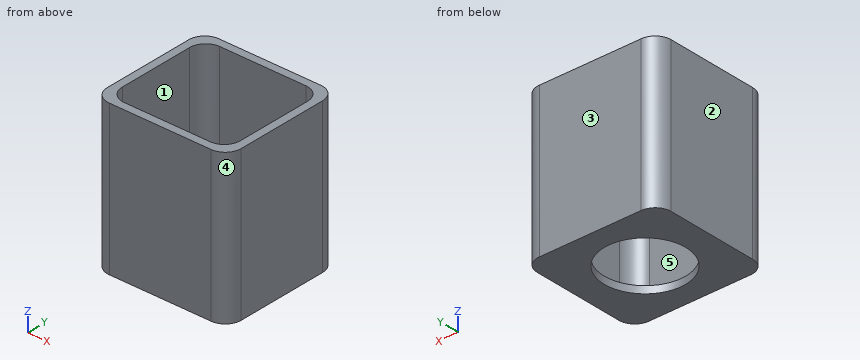
```python
from build123d import *

# Parameters (mm, degrees)
F0_W     = 42
F0_H     = 39
F0_R     = 12.75
F1_DEPTH = 47.25
F2_W     = 37
F2_H     = 34
F2_R     = 12.75
F3_DEPTH = 45
F4_R     = 5


with BuildPart() as f1:
    # F0 (on Top) → F1 (new body)
    with BuildSketch(Plane.XY):
        Rectangle(F0_W, F0_H)
        Circle(F0_R, mode=Mode.SUBTRACT)
    extrude(amount=F1_DEPTH)

    # F2 (on face) → F3 (cut)
    with BuildSketch(Plane.XY.offset(47.25)):
        Rectangle(F2_W, F2_H)
        Circle(F2_R, mode=Mode.SUBTRACT)
    extrude(amount=-F3_DEPTH, mode=Mode.SUBTRACT)

    # F4
    f4_edges = [f1.edges().sort_by_distance(p)[0] for p in [
        (-21, -19.5, 23.625),
        (21, -19.5, 23.625),
        (21, 19.5, 23.625),
        (-21, 19.5, 23.625),
        (-18.5, -17, 24.75),
        (-18.5, 17, 24.75),
        (18.5, 17, 24.75),
        (18.5, -17, 24.75),
    ]]
    fillet(f4_edges, radius=F4_R)


solid = f1.part
```
Geometry: final body of the model. Coordinates: model frame, mm. Face numbers are marked on the shaded views. A direction names the side the tool comes from. Coordinates: 2 decimals unless noted, no trailing zeros. Order: outer loops, then holes, each group sorted by start corner. A loop starts at its lowest first (then second) coordinate and runs counter-clockwise, first axis right, second up. Notation, with made-up numbers: (-4.5, 30) - (30.5, 30) arc R22 cw to (30.5, 59) - close; hole circle Ø6 at (84.5, 51.25). An arc over 180 degrees is marked (long way). Write each question's results on one line, items separated by ' | '.
1) Set-up query: the marked faces 4 and 5. Return all of +Z, -Z, +X, -X, +Y, -Y with unobstructed straight access to the full face (end or side cutting, diameter ignored); none if empty.
Results list:
face 4: +Z, -Z, +X, -Y | face 5: +Z
2) Pin query (flat end, axial travel): pin 1 (5 mm diameter, centred on x = 13.5, y = 7.5, fed in from +Z). Return the tip coordinate at first contact, or that it passes through.
Results list:
pin 1: z = 2.25
3) Pull-direction query (Y, two-part tool) for the marked faces 1, 2 and 3; classes: pulls with the +Y half, pulls with the -Y half, needs draft (parallel to the pull), parting line crosses it, or undercut.
Results list:
face 1: undercut | face 2: needs draft | face 3: pulls with the +Y half
4) Section B-B, the plane x = 0. Return loops of the section in (y, z), plus the area to 3 significant figures.
Results list:
outline: (-19.5, 0) - (-12.75, 0) - (-12.75, 2.25) - (-17, 2.25) - (-17, 47.25) - (-19.5, 47.25) - close; (12.75, 0) - (19.5, 0) - (19.5, 47.25) - (17, 47.25) - (17, 2.25) - (12.75, 2.25) - close | area: 255 mm^2
5) Line query: line 1 (X direction, y = 11, z = 27.5); line 2 (Y direction, x = -4.5, z = 19); line 3 (Y direction, x = 0, z = 0.7). Output: solid intervals per line, ascending. Write a range as from..to.
Results list:
line 1: -21..-18.5, 18.5..21 | line 2: -19.5..-17, 17..19.5 | line 3: -19.5..-12.75, 12.75..19.5
6) Section A-A, the plane y = 0. Return loops of the section in (x, z).
Results list:
outline: (-21, 0) - (-12.75, 0) - (-12.75, 2.25) - (-18.5, 2.25) - (-18.5, 47.25) - (-21, 47.25) - close; (12.75, 0) - (21, 0) - (21, 47.25) - (18.5, 47.25) - (18.5, 2.25) - (12.75, 2.25) - close
7) Section C-C, the plane z = 6. Return loops of the section in (x, y).
Results list:
outline: (-21, -14.5) arc R5 ccw to (-16, -19.5) - (16, -19.5) arc R5 ccw to (21, -14.5) - (21, 14.5) arc R5 ccw to (16, 19.5) - (-16, 19.5) arc R5 ccw to (-21, 14.5) - close; hole (-18.5, -12) arc R5 ccw to (-13.5, -17) - (13.5, -17) arc R5 ccw to (18.5, -12) - (18.5, 12) arc R5 ccw to (13.5, 17) - (-13.5, 17) arc R5 ccw to (-18.5, 12) - close
